from build123d import *

# Parameters (mm, degrees)
SKETCH1_W           = 1150
SKETCH1_H           = 34
BOSS_EXTRUDE1_DEPTH = 1950
CUT_EXTRUDE3_DEPTH  = 1950
CUT_EXTRUDE4_DEPTH  = 1950
SKETCH4_W           = 238.582936687
SKETCH4_H           = 386.127647534
BOSS_EXTRUDE5_DEPTH = 35


with BuildPart() as part:
    # Sketch1 → Boss-Extrude1 (new body)
    with BuildSketch(Plane(origin=(0, 0, 0), x_dir=(0, 0, -1), z_dir=(1, 0, 0))):
        Rectangle(SKETCH1_W, SKETCH1_H)
    extrude(amount=BOSS_EXTRUDE1_DEPTH)

    # Sketch2 → Cut-Extrude3 (cut)
    with BuildSketch(Plane(origin=(1950, 0, 0), x_dir=(0, 0, -1), z_dir=(1, 0, 0))):
        with BuildLine():
            Line((454.506922221, 17), (575, 17))
            Line((575, 17), (575, -17))
            add(Edge.make_bspline(
                [(489.682610702, -2.777028038), (534.776362322, 4.522431825), (575, -17)],
                knots=[0, 0, 0, 1, 1, 1], degree=2))
            add(Edge.make_bspline(
                [(454.506922221, 17), (483.149171875, 14.577610521), (489.682610702, -2.777028038)],
                knots=[0, 0, 0, 0.737774991, 0.737774991, 0.737774991], degree=2))
        make_face()
        with BuildLine():
            Line((-454.506922221, 17), (-575, 17))
            Line((-575, 17), (-575, -17))
            add(Edge.make_bspline(
                [(-489.682610702, -2.777028038), (-534.776362322, 4.522431825), (-575, -17)],
                knots=[0, 0, 0, 1, 1, 1], degree=2))
            add(Edge.make_bspline(
                [(-454.506922221, 17), (-483.149171875, 14.577610521), (-489.682610702, -2.777028038)],
                knots=[0, 0, 0, 0.737774991, 0.737774991, 0.737774991], degree=2))
        make_face()
    extrude(amount=-CUT_EXTRUDE3_DEPTH, mode=Mode.SUBTRACT)

    # Sketch3 → Cut-Extrude4 (cut)
    with BuildSketch(Plane.XZ.offset(17)):
        with BuildLine():
            Line((1800, 575), (1950, 575))
            Line((1950, 575), (1950, 195))
            add(Edge.make_bspline(
                [(1950, 195), (1676.162586963, 312.417807061), (1800, 575)],
                knots=[0, 0, 0, 1, 1, 1], degree=2))
        make_face()
        with BuildLine():
            Line((1950, -195), (1950, -575))
            Line((1950, -575), (1800, -575))
            add(Edge.make_bspline(
                [(1950, -195), (1676.162586963, -312.417807061), (1800, -575)],
                knots=[0, 0, 0, 1, 1, 1], degree=2))
        make_face()
    extrude(amount=-CUT_EXTRUDE4_DEPTH, mode=Mode.SUBTRACT)

    # Sketch4 → Boss-Extrude5 (add)
    with BuildSketch(Plane(origin=(0, 17, 0), x_dir=(1, 0, 0), z_dir=(0, 1, 0))):
        with Locations((1708.01468048, 0)):
            Rectangle(SKETCH4_W, SKETCH4_H)
    extrude(amount=BOSS_EXTRUDE5_DEPTH)


solid = part.part
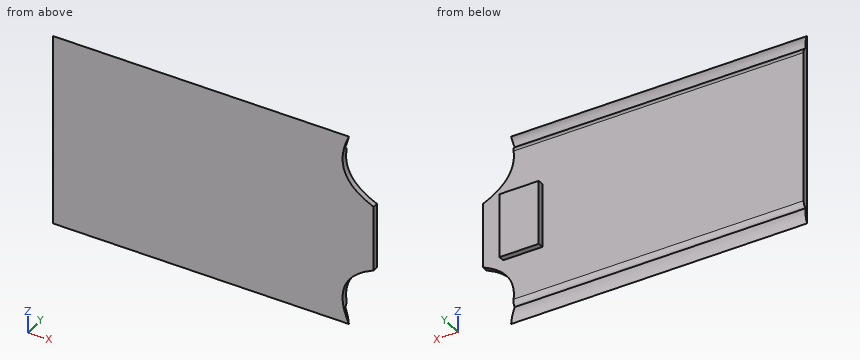
Read the model definition and answer for the solid it produces. Units are mm, in the model's axes. Give positions to 0.01 mm unless a question says otherwise; leave off trailing zeros. Write each loop counter-clockwise with the first axis right and the second up, starting at its lowest first coordinate (ties: lowest second). Pieces come first, ordered by that corner, then holes. Notation, with made-up numbers: (37.5, 24) -> (90.5, 24) arc R15 cw to (90.5, 49) -> close; hole circle Ø4 at (-8, 86.25). An arc over 180 degrees is marked (long way). Answer as a JSON object with one key per item and string values. Group by question number.
1) Consider L1, parallel to Y at x = 191, z = 504; L2, parallel to X at y = 44.5, z = -46.5; L3, parallel to Y at x = 687, z = 438.5. Determine where each line is inside the solid, lowest interval first. Write a range as from..to.
2) Find section B-B (y = 38). Write down the section's boundary in (x, z).
3) Each of these flat-tipped pins is pushed along its axis until it touches: P1, Ø10, axis at x = 817.5, y = -9.5, coming from the +Z side; P2, Ø17.5, axis at y = 33.5, z = 27.5, coming from the -X side; P3, Ø8, axis at y = 32.5, z = -103.5, coming from the +X side; P4, Ø6, axis at y = -7.5, z = 3, coming from the -X side. Where does it stop, or does it pass through?
4) Find section A-A (z = 66). Write down the section's boundary in (x, y).
Values follow:
{
 "1": {"L1": "y = -17..-1.18", "L2": "x = 1588.72..1827.31", "L3": "y = -17..17"},
 "2": {"outline": "(1588.72, -193.06) -> (1827.31, -193.06) -> (1827.31, 193.06) -> (1588.72, 193.06) -> close"},
 "3": {"P1": "stops at z = 570.11", "P2": "stops at x = 1588.72", "P3": "stops at x = 1827.31", "P4": "stops at x = 0"},
 "4": {"outline": "(0, -17) -> (1950, -17) -> (1950, 17) -> (1827.31, 17) -> (1827.31, 52) -> (1588.72, 52) -> (1588.72, 17) -> (0, 17) -> close"}
}
